Input: part model. Units: mm. Frame: model coordinates. A direction names the side the tool comes from. Give positions to 0.01 mm unless a question says otherwise; leave off trailing zeros. Loops run counter-clockwise (first coordinate to the right, second up) from the corner with the lowest first, then second, coordinate; pieces in that order, holes last. Notation, with made-up numbers: M 10.25,55 L 23.25,55 A5 ccw 23.25,60 Z; hole C 82.25,-32 d5. An arc over 180 degrees is marked long. Answer as a JSON object with one key per item and string values. Group by question number.
1) Access query for faces 1 (the cylindrical face through (106.33, 1.5, -0.69)), 2 (the cylindrical face through (68, 6, 3)). Directions: +Z, -Z, +X, -X, +Y, -Y. A direction counts if a zero-diameter tool reaches every point of the face in a straight line with its end or side. Return the directions, or none.
2) Draft query along Z for faces 3 (the cylindrical face through (-1.38, 8.5, -33.58)), 4 (the cylindrical face through (-106.18, 8.5, -0.27)), 5 (the cylindrical face through (-68.31, 5.94, 1.92)), 6 (the flat face through (-2, 10, -5)). Return one class per face: +Z half, -Z half, draft (parallel to the pull), parting line (faces both ways), or undercut.
3) Section query B-B on y = 7.5. Return loops of the section in (x, z).
4) Ray query, L1, parallel to Z at x = 33, y = 4.5; L2, parallel to X at y = 2.25, z = -19; L3, parallel to X at y = 2.75, z = 13. Return the intervals inside material, ascending.
5) First-contact query: P1, Ø1.5, axis at x = 12.5, y = 2, coming from the +Z side; P2, Ø4.5, axis at x = 71, z = -12.5, coming from the +Y side; P3, Ø1.2, axis at x = 70.5, z = 4, coming from the +Y side; P4, Ø6, axis at y = 4.5, z = -3.5, coming from the +X side. Flat tips, straight axial feed; report the tip coordinate or a pass-through.
from build123d import *

# Parameters (mm, degrees)
BOSS_EXTRUDE1_DEPTH = 10
FILLET1_R           = 5
CUT_EXTRUDE7_START  = -2
SKETCH5_R           = 2
CUT_EXTRUDE7_DEPTH  = 8


with BuildPart() as part:
    # Sketch1 → Boss-Extrude1 (new body)
    with BuildSketch(Plane(origin=(0, 0, 0), x_dir=(1, 0, 0), z_dir=(0, 1, 0))):
        with BuildLine():
            Line((-112.915113285, 15), (-102.291556109, -15))
            ThreePointArc((-102.291556109, -15), (-96.809111593, -22.242520439), (-88.151933742, -24.992897111))
            Line((-88.151933742, -24.992897111), (88.151933742, -24.992897111))
            ThreePointArc((88.151933742, -24.992897111), (96.809111593, -22.242520439), (102.291556109, -15))
            Line((102.291556109, -15), (112.915113285, 15))
            ThreePointArc((112.915113285, 15), (111.025114246, 28.664280739), (98.775490918, 35.007102889))
            Line((98.775490918, 35.007102889), (-98.775490918, 35.007102889))
            ThreePointArc((-98.775490918, 35.007102889), (-111.025114246, 28.664280739), (-112.915113285, 15))
        make_face()
    extrude(amount=BOSS_EXTRUDE1_DEPTH)

    # Fillet1
    fillet1_edges = [part.edges().sort_by_distance(p)[0] for p in [
        (0, 0, -35.007102889),
        (111.025114246, 0, -28.664280739),
        (107.603334697, 0, 0),
        (96.809111593, 0, 22.242520439),
        (0, 10, -35.007102889),
        (-111.025114246, 10, -28.664280739),
        (-107.603334697, 10, 0),
        (-96.809111593, 10, 22.242520439),
        (0, 10, 24.992897111),
        (0, 0, 24.992897111),
        (107.603334697, 10, 0),
        (-107.603334697, 0, 0),
    ]]
    fillet(fillet1_edges, radius=FILLET1_R - 0.0001)  # a hair under: the kernel refuses the full size

    # Sketch5 → Cut-Extrude7 (cut)
    with BuildSketch(Plane.XZ.offset(CUT_EXTRUDE7_START)):
        with Locations(Location((-70, 2.992897111, 0), (0, 0, 270))):
            Circle(SKETCH5_R)
        with Locations(Location((-70, -13.007102889, 0), (0, 0, 90))):
            Circle(SKETCH5_R)
        with Locations(Location((70, -13.007102889, 0), (0, 0, 270))):
            Circle(SKETCH5_R)
        with Locations(Location((70, 2.992897111, 0), (0, 0, 90))):
            Circle(SKETCH5_R)
    extrude(amount=-CUT_EXTRUDE7_DEPTH, mode=Mode.SUBTRACT)


solid = part.part
Output:
{
 "1": {"face 1": "+Z, +X, -Y", "face 2": "+Y"},
 "2": {"face 3": "-Z half", "face 4": "+Z half", "face 5": "undercut", "face 6": "draft"},
 "3": {"outline": "M -112.28,-15.22 A14.33 ccw -98.78,-34.34 L 98.78,-34.34 A14.33 ccw 112.28,-15.22 L 101.66,14.78 A14.33 ccw 88.15,24.32 L -88.15,24.32 A14.33 ccw -101.66,14.78 Z; hole C -70,-13.01 d4; hole C -70,2.99 d4; hole C 70,-13.01 d4; hole C 70,2.99 d4"},
 "4": {"L1": "z = -34.98 to 24.97", "L2": "x = -112.92 to 112.92", "L3": "x = -102.43 to 102.43"},
 "5": {"P1": "stops at z = 24.46", "P2": "stops at y = 10", "P3": "stops at y = 2", "P4": "stops at x = 109.9"}
}
